from build123d import *

# Parameters (mm, degrees)
SKETCH1_W               = 76.2
SKETCH1_H               = 50.8
BOSS_EXTRUDE1_DEPTH     = 6.35
CAVITY5_OUTLINE_R       = 18.161
CAVITY5_OUTLINE_R_2     = 1.5875
CAVITY5_DEPTH           = 6.35
SKETCH3_R               = 1.5875
CUT_EXTRUDE1_DEPTH      = 92.800885072
MIRROR2_COPY_1_SKETCH_R = 1.5875
MIRROR2_COPY_1_DEPTH    = 92.800885072
SKETCH4_R               = 1.5875
CUT_EXTRUDE2_DEPTH      = 92.800885072


# Read off the part's stored shape, not the designer's step: Cavity5
with BuildPart() as part:
    # Sketch1 → Boss-Extrude1 (new body)
    with BuildSketch(Plane.XY):
        with Locations((38.1, 25.4)):
            Rectangle(SKETCH1_W, SKETCH1_H)
    extrude(amount=BOSS_EXTRUDE1_DEPTH)

    # Cavity5 outline → Cavity5 (cut)
    with BuildSketch(Plane.XY):
        with Locations((38.1, 25.4)):
            Circle(CAVITY5_OUTLINE_R)
        with Locations((16.188175065, 25.4)):
            Circle(CAVITY5_OUTLINE_R_2)
        with Locations((60.011824935, 25.4)):
            Circle(CAVITY5_OUTLINE_R_2)
    extrude(amount=CAVITY5_DEPTH, mode=Mode.SUBTRACT)

    # Sketch3 → Cut-Extrude1 (cut, through all)
    with BuildSketch(Plane(origin=(0, 0, 0), x_dir=(-1, 0, 0), z_dir=(0, 0, -1))):
        with Locations((-68.2625, 44.45)):
            Circle(SKETCH3_R)
    cut_extrude1 = extrude(amount=-CUT_EXTRUDE1_DEPTH, mode=Mode.SUBTRACT)

    # Mirror1: Cut-Extrude1 across plane
    add(cut_extrude1.mirror(Plane(origin=(38.1, 0, 0), x_dir=(0, 0, 1), z_dir=(1, 0, 0))), mode=Mode.SUBTRACT)

    # Mirror2: Cut-Extrude1 across plane
    add(cut_extrude1.mirror(Plane.ZX.offset(25.4)), mode=Mode.SUBTRACT)

    # Mirror2 copy 1 sketch → Mirror2 copy 1 (cut, through all)
    with BuildSketch(Plane(origin=(76.2, 50.8, 0), x_dir=(1, 0, 0), z_dir=(0, 0, -1))):
        with Locations((-68.2625, 44.45)):
            Circle(MIRROR2_COPY_1_SKETCH_R)
    extrude(amount=-MIRROR2_COPY_1_DEPTH, mode=Mode.SUBTRACT)

    # Sketch4 → Cut-Extrude2 (cut, through all)
    with BuildSketch(Plane(origin=(0, 0, 0), x_dir=(-1, 0, 0), z_dir=(0, 0, -1))):
        with Locations((-19.05, 44.45)):
            Circle(SKETCH4_R)
        with Locations((-57.15, 44.45)):
            Circle(SKETCH4_R)
        with Locations((-57.15, 6.35)):
            Circle(SKETCH4_R)
        with Locations((-19.05, 6.35)):
            Circle(SKETCH4_R)
    extrude(amount=-CUT_EXTRUDE2_DEPTH, mode=Mode.SUBTRACT)


solid = part.part
Part model, mm, in its own coordinate system. Round coordinates to 2 decimals unless told otherwise and drop trailing zeros. Loops run counter-clockwise (first coordinate to the right, second up) from the corner with the lowest first, then second, coordinate; pieces in that order, holes last. Notation, with made-up numbers: (43, -17.5) - (68, -17.5) arc R16 cw to (68, -4.5) - close; hole circle Ø1 at (46, 17.5). An arc over 180 degrees is marked (long way). Answer as a JSON object with one key per item and string values.
Item 1: Band-saw the part on C-C on z = 4. State how many separate pieces and enclosed holes the cut face has, plus the area to 3 significant figures.
Output:
{"separate pieces": "1", "enclosed holes": "11", "area": "2,760 mm2"}
Item 2: Pull direction X, two halves, no side cores. Call faces 1 (the face through (76.2, 25, 3)), 2 (the face through (58.41, 5.384, 3.131)), 3 (the face through (20.6, 31.4, 0)): pulls with the +X half, pulls with the -X half, needs draft (parallel to the pull), parting line crosses it, or undercut.
Output:
{"face 1": "pulls with the +X half", "face 2": "undercut", "face 3": "needs draft"}
Item 3: Band-saw the part on B-B on y = 25.4. List the corners of the cut face in (x, z), plus the area to 3 significant figures.
Output:
{"outline": "(0, 0) - (14.6, 0) - (14.6, 6.35) - (0, 6.35) - close; (17.78, 0) - (19.94, 0) - (19.94, 6.35) - (17.78, 6.35) - close; (56.26, 0) - (58.42, 0) - (58.42, 6.35) - (56.26, 6.35) - close; (61.6, 0) - (76.2, 0) - (76.2, 6.35) - (61.6, 6.35) - close", "area": "213 mm2"}
Item 4: Band-saw the part on D-D on x = 19.05. List the corners of the cut face in (y, z).
Output:
{"outline": "(0, 0) - (4.76, 0) - (4.76, 6.35) - (0, 6.35) - close; (7.94, 0) - (42.86, 0) - (42.86, 6.35) - (7.94, 6.35) - close; (46.04, 0) - (50.8, 0) - (50.8, 6.35) - (46.04, 6.35) - close"}
Item 5: Band-saw the part on A-A on x = 38.1. List the corners of the cut face in (y, z).
Output:
{"outline": "(0, 0) - (7.24, 0) - (7.24, 6.35) - (0, 6.35) - close; (43.56, 0) - (50.8, 0) - (50.8, 6.35) - (43.56, 6.35) - close"}
Item 6: Wall check: L1, parallel to Y at x = 57, z = 1.75; L2, parallel to Y at x = 38.1, z = 1.75; L3, parallel to Y at x = 18.5, z = 3.75. Give the ranges that are in metal, low to high.
Output:
{"L1": "0 to 4.77, 7.93 to 42.87, 46.03 to 50.8", "L2": "0 to 7.24, 43.56 to 50.8", "L3": "0 to 4.86, 7.84 to 42.96, 45.94 to 50.8"}
